Part model, mm, in its own coordinate system. A direction names the side the tool comes from. Round coordinates to 2 decimals unless told otherwise and drop trailing zeros. Write each loop counter-clockwise with the first axis right and the second up, starting at its lowest first coordinate (ties: lowest second). Pieces come first, ordered by that corner, then holes. Notation, with made-up numbers: (17.5, -33) -> (62.5, -33) arc R14 cw to (62.5, -17) -> close; hole circle Ø3 at (45.5, -26). An arc over 180 degrees is marked (long way). Return JSON: item names as keys, results as strings. Group by question number.
```python
from build123d import *

# Parameters (mm, degrees)
F1_DEPTH = 12
F2_R     = 3
F3_DEPTH = 50.001
F4_R     = 5


with BuildPart() as f1:
    # F0 (on Top) → F1 (new body)
    with BuildSketch(Plane.XY):
        Polygon((-17.527781, 97.694382), (-30.027781, 97.694382), (-30.027781, -172.305618), (-17.527781, -172.305618), (-17.527781, -159.305618), (7.472219, -159.305618), (7.472219, -172.305618), (19.972219, -172.305618), (19.972219, 97.694382), (7.472219, 97.694382), (7.472219, 82.484039), (-17.527781, 82.484039), align=None)
    extrude(amount=F1_DEPTH)

    # F2 (on face) → F3 (cut, through all)
    with BuildSketch(Plane(origin=(-30.027781, 0, 0), x_dir=(0, -1, 0), z_dir=(-1, 0, 0))):
        with Locations((-91.194382, 6)):
            Circle(F2_R)
        with Locations((165.805618, 6)):
            Circle(F2_R)
    extrude(amount=-F3_DEPTH, mode=Mode.SUBTRACT)

    # F4
    f4_edges = [f1.edges().sort_by_distance(p)[0] for p in [
        (-23.777781, 97.694382, 12),
        (-23.777781, 97.694382, 0),
        (13.722219, 97.694382, 12),
        (13.722219, 97.694382, 0),
        (-23.777781, -172.305618, 12),
        (13.722219, -172.305618, 12),
        (-23.777781, -172.305618, 0),
        (13.722219, -172.305618, 0),
    ]]
    fillet(f4_edges, radius=F4_R)


solid = f1.part
```
Item 1: Wall check: L1, parallel to Y at x = 5.5, z = 2.75; L2, parallel to Y at x = 17.5, z = 3.5; L3, parallel to Y at x = 12, z = 2.5. Give the ranges that are in metal, low to high.
Item 2: Which spindle directions (+Z, -Z, +X, -X, +Y, -Y) get a long thin tool onto all of the face, cutting with end or side? Do faces 1 (the face through (-17.528, -164, 3)), 2 (the face through (13.635, 96.191, 1.426)), 3 (the face through (-17.528, 88, 7)). Say none if no direction does.
Item 3: Two-plate mould, pull along Z, no slides. Class faces 4 (the face through (-23.865, 88.333, 6.901)), 5 (the face through (-23.69, -170.802, 10.574)), 6 (the face through (-30.028, -35, 6)): released by +Z, released by -Z, zero draft, split by the parting line, or undercut.
Item 4: Flat gauge pins, fed straight in: P1, Ø4, axis at x = -10.5, z = 1.5, coming from the +Y side; P2, Ø12, axis at x = -2, y = 2.5, coming from the -Z side. Where does each tip first touch, or does it go through?
Item 5: Cut at A-A (x = -25). Write the cut outline in (y, z).
Item 6: Cut at B-B (x = 1). Write the cut outline in (y, z), then the cut area to 3 significant figures.
Checks:
{
 "1": {"L1": "y = -159.31 to 82.48", "L2": "y = -172.08 to -167.46, -164.15 to 89.54, 92.85 to 97.46", "L3": "y = -171.64 to 97.02"},
 "2": {"face 1": "+Z, -Z, -Y", "face 2": "-Z, +X, -X, +Y", "face 3": "+Z, -Z, +Y"},
 "3": {"face 4": "undercut", "face 5": "released by +Z", "face 6": "zero draft"},
 "4": {"P1": "stops at y = 82.48", "P2": "stops at z = 0"},
 "5": {"outline": "(-172.31, 5) arc R5 ccw to (-167.31, 0) -> (92.69, 0) arc R5 ccw to (97.69, 5) -> (97.69, 7) arc R5 ccw to (92.69, 12) -> (-167.31, 12) arc R5 ccw to (-172.31, 7) -> close; hole circle Ø6 at (-165.81, 6); hole circle Ø6 at (91.19, 6)"},
 "6": {"outline": "(-159.31, 0) -> (82.48, 0) -> (82.48, 12) -> (-159.31, 12) -> close", "area": "2,900 mm2"}
}
